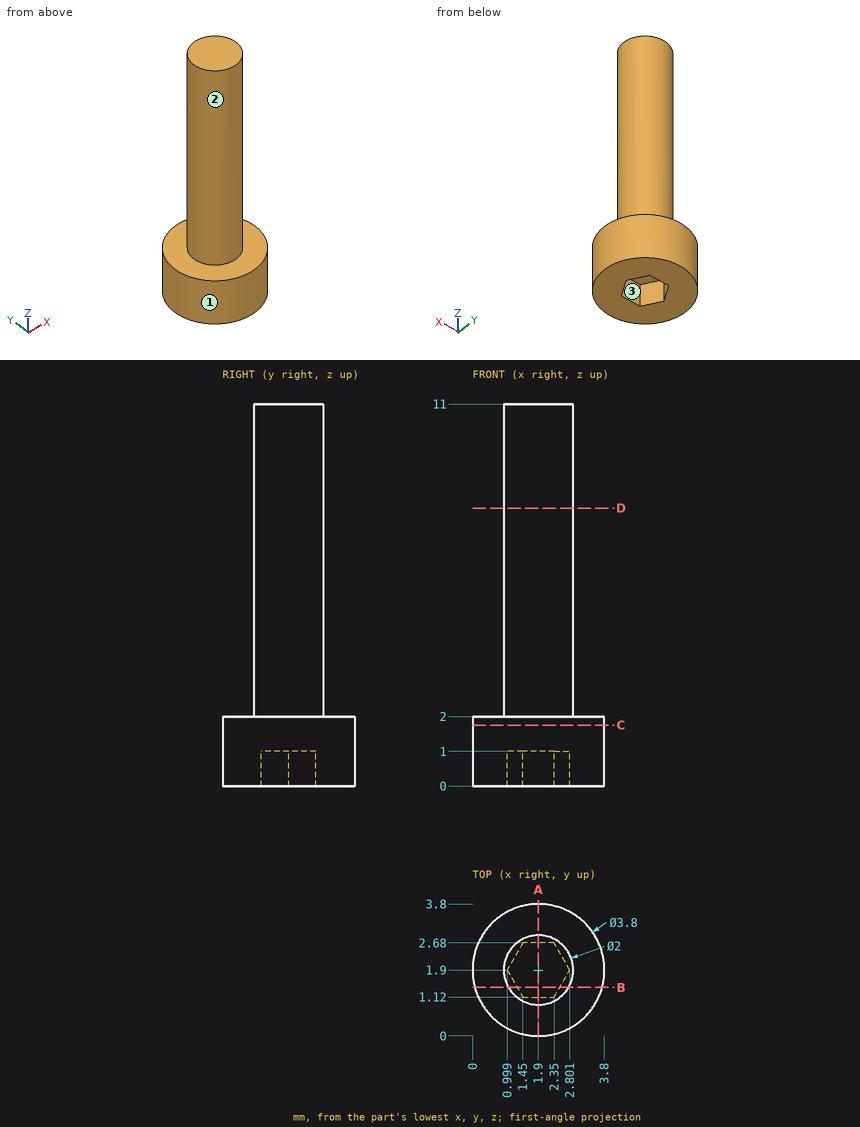
Answer from the drawing. Dimensions are ordinates in mm from the lowest x, y and z of the part. A direction names the side the tool comes from. Round coordinates to 2 decimals unless told otherwise and drop trailing zeros. Order: outer loops, then holes, each group sorted by start corner. A loop starts at its lowest first (then second) coordinate and runs counter-clockwise, first axis right, second up.
1) For the marked faces 1, 2 and 3, determine the directions among +Z, -Z, +X, -X, +Y, -Y from which every point of the face is accessible in a straight line to the end or side of a thin tool.
2) The part is cut by section C-C on z = 1.75. Write down the section's boundary in (x, y).
3) The part is cut by section B-B on y = 1.4. Write down the section's boundary in (x, z), plus the area to 3 significant figures.
4) The part is cut by section A-A on x = 1.9. Write down the section's boundary in (y, z).
5) Flat-ended cylindrical pins translate along their axes: pin 1 (1.5 mm diameter, centred on y = 3, z = 5.5, fed in from +X); pin 2 (1.5 mm diameter, centred on y = 1, z = 2.5, fed in from +X). Find the tip coordinate at first contact, or state that the pin passes through.
6) Straight lines are drawn through the part: L1, parallel to Z at x = 1.25, y = 1.8; L2, parallel to Z at x = 0.2, y = 1.3; L3, parallel to X at y = 1.5, z = 8.5. For each, find the intervals that lie inside material, in ascending order.
7) The part is cut by section D-D on z = 8. Write down the section's boundary in (x, y).
Resolved:
1. face 1: +Z, -Z
1. face 2: +Z
1. face 3: -Z
2. outline: circle Ø3.8 at (1.9, 1.9)
3. outline: (0.07, 0) - (1.29, 0) - (1.29, 1) - (2.51, 1) - (2.51, 0) - (3.73, 0) - (3.73, 2) - (2.77, 2) - (2.77, 11) - (1.03, 11) - (1.03, 2) - (0.07, 2) - close
3. area: 21.7 mm2
4. outline: (0, 0) - (1.12, 0) - (1.12, 1) - (2.68, 1) - (2.68, 0) - (3.8, 0) - (3.8, 2) - (2.9, 2) - (2.9, 11) - (0.9, 11) - (0.9, 2) - (0, 2) - close
5. pin 1: stops at x = 2.84
5. pin 2: stops at x = 3.77
6. L1: z = 1 to 11
6. L2: z = 0 to 2
6. L3: x = 0.98 to 2.82
7. outline: circle Ø2 at (1.9, 1.9)
